from build123d import *

# Parameters (mm, degrees)
F1_DEPTH = 15.875


with BuildPart() as f1:
    # F0 (on Top) → F1 (new body)
    with BuildSketch(Plane.XY):
        Polygon((209.55, -374.65), (209.55, -425.45), (476.25, -425.45), (476.25, -374.65), (495.3, -374.65), (495.3, -184.260472), (476.25, -184.260472), (476.25, -133.460472), (495.3, -133.460472), (495.3, 374.65), (476.25, 374.65), (476.25, 406.4), (425.45, 406.4), (425.45, 425.45), (-63.610472, 425.45), (-63.610472, 406.4), (-114.410472, 406.4), (-114.410472, 425.45), (-444.5, 425.45), (-444.5, 406.4), (-495.3, 406.4), (-495.3, 139.7), (-444.5, 139.7), (-444.5, 120.65), (-114.410472, 120.65), (-114.410472, 139.7), (-81.119703, 139.7), (-57.579575, 116.159872), (-71.04996, 102.689488), (172.539488, -140.89996), (186.009872, -127.429575), (209.55, -150.969703), (209.55, -184.260472), (190.5, -184.260472), (190.5, -374.65), align=None)
    extrude(amount=F1_DEPTH)


solid = f1.part
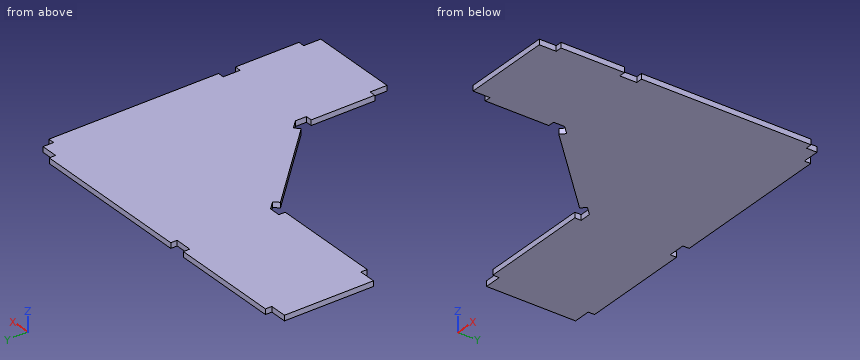
Part model, mm, in its own coordinate system. Give positions to 0.01 mm unless a question says otherwise; leave off trailing zeros. Order: outer loops, then holes, each group sorted by start corner. A loop starts at its lowest first (then second) coordinate and runs counter-clockwise, first axis right, second up. Notation, with made-up numbers: (13, -28) -> (26, -28) arc R19 ccw to (26, -3) -> close; hole circle Ø7 at (88.5, 78.25). An arc over 180 degrees is marked (long way). Use one line per item in the form item = value.
(1) Flat gauge pins, fed straight in: P1, Ø5, axis at x = -94.5, z = 7, coming from the +Y side; P2, Ø8, axis at y = 417.5, z = 11, coming from the +X side; P3, Ø8, axis at x = 488.5, z = 7.5, coming from the +Y side. Where does each tip first touch, or does it go through?
Solution:
P1 = 406.4
P2 = 425.45
P3 = 374.65
(2) Drill centre lines: line 1 (Y direction, x = -170.5, z = 11.5); line 2 (Y direction, x = -106.5, z = 14.75); line 3 (X direction, y = -347, z = 12). Where is each one in solid material? Low to high. Write a range as from..to.
Solution:
line_1 = 120.65..425.45
line_2 = 139.7..406.4
line_3 = 190.5..495.3
(3) Saw through at A-A (y = -256). Write the cut outline in (x, z) (3 decimals).
Solution:
outline = (190.5, 0) -> (495.3, 0) -> (495.3, 15.875) -> (190.5, 15.875) -> close
(4) Saw through at B-B (x = -354). Write the cut outline in (y, z) (3 decimals).
Solution:
outline = (120.65, 0) -> (425.45, 0) -> (425.45, 15.875) -> (120.65, 15.875) -> close
